Answer from the drawing. Dimensions are ordinates in mm from the lowest x, y and z of the part. Coordinates: 2 decimals unless noted, no trailing zeros. Loops run counter-clockwise (first coordinate to the right, second up) from the corner with the lowest first, then second, coordinate; pieces in that order, holes last. Notation, with made-up numbers: (-12.5, 48) - (30.5, 48) arc R32 ccw to (30.5, 75) - close; hole circle Ø1 at (-1, -14.5). An arc over 180 degrees is marked (long way). Write each question's results on one line, items separated by ' | '. Start each with the question number.
1. A cutting plane is placed at B-B on z = 0.5. Determine the outline of the cut face in (x, y) (1 decimal).
2. Each of these flat-tipped pins is pushed along its axis until it touches: P1, Ø1.5, axis at x = 3.5, y = 6, coming from the -Z side; P2, Ø1.5, axis at x = 7, z = 4, coming from the +Y side. Where does it stop, or does it pass through?
3. Find the intervals of material crossed by line 1 along Y through (x, z) = (6.75, 6) (1 decimal); line 2 along Y through (x, z) = (2.75, 4.25) (1 decimal); line 3 along X through (y, z) = (2.5, 1.5), in increasing order. Write a range as [from, to].
4. A cutting plane is placed at A-A on y = 3. Determine the outline of the cut face in (x, z).
5. A cutting plane is placed at C-C on x = 5. Determine the outline of the cut face in (y, z).
6. A cutting plane is placed at D-D on x = 9. Determine the outline of the cut face in (y, z), then the cut area to 3 significant figures.
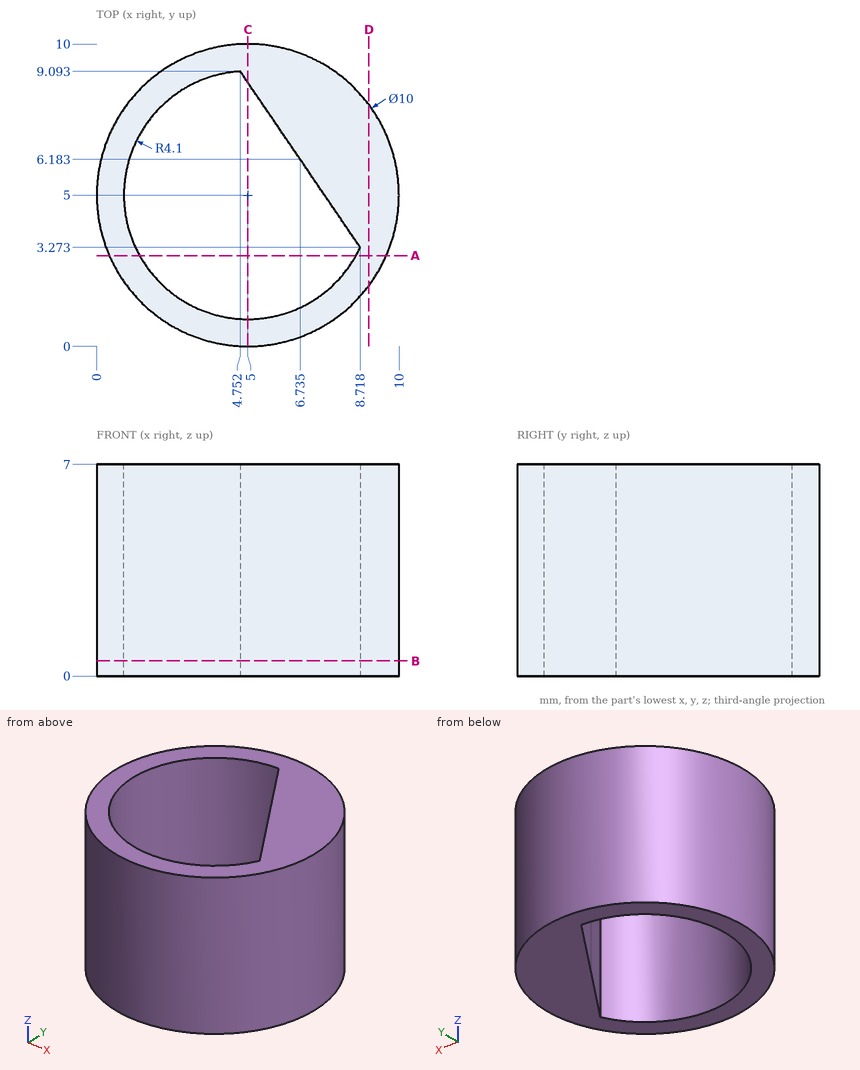
Values:
1) outline: circle Ø10 at (5, 5); hole (1.6, 2.7) arc R4.1 ccw to (8.7, 3.3) - (6.7, 6.2) - (4.8, 9.1) arc R4.1 ccw to start
2) P1: through | P2: y = 9.84
3) line 1: [0.3, 1.3], [6.2, 9.7] | line 2: [0.5, 1.6], [8.4, 9.5] | line 3: [0.67, 1.75], [8.25, 9.33]
4) outline: (0.42, 0) - (1.42, 0) - (1.42, 7) - (0.42, 7) - close; (8.58, 0) - (9.58, 0) - (9.58, 7) - (8.58, 7) - close
5) outline: (0, 0) - (0.9, 0) - (0.9, 7) - (0, 7) - close; (8.73, 0) - (10, 0) - (10, 7) - (8.73, 7) - close
6) outline: (2, 0) - (8, 0) - (8, 7) - (2, 7) - close | area: 42.0 mm^2
